from build123d import *

# Parameters (mm, degrees)
ESQUISSE1_W             = 8
ESQUISSE1_H             = 59
BOSS_EXTRU_1_DEPTH      = 60
ESQUISSE3_R             = 30
ESQUISSE3_R_2           = 29
BOSS_EXTRU_2_DEPTH      = 60
ESQUISSE4_R             = 29
ENL_V_MAT_EXTRU_3_DEPTH = 30
ENL_V_MAT_EXTRU_5_DEPTH = 1.5
ESQUISSE6_R             = 29
ENL_V_MAT_EXTRU_6_DEPTH = 22
ESQUISSE7_R             = 2
ENL_V_MAT_EXTRU_7_DEPTH = 6.5
ESQUISSE9_R             = 0.5
ENL_V_MAT_EXTRU_8_DEPTH = 4


with BuildPart() as part:
    # Esquisse1 → Boss.-Extru.1 (new body)
    with BuildSketch(Plane.XY):
        with Locations((4, 29.5)):
            Rectangle(ESQUISSE1_W, ESQUISSE1_H)
    extrude(amount=BOSS_EXTRU_1_DEPTH)

    # Esquisse3 → Boss.-Extru.2 (add)
    with BuildSketch(Plane(origin=(0, 0, 0), x_dir=(-1, 0, 0), z_dir=(0, 0, -1))):
        with Locations((-4, 29.5)):
            Circle(ESQUISSE3_R)
        with Locations((-4, 29.5)):
            Circle(ESQUISSE3_R_2, mode=Mode.SUBTRACT)
    extrude(amount=-BOSS_EXTRU_2_DEPTH)

    # Esquisse4 → Enlèv. mat.-Extru.3 (cut)
    with BuildSketch(Plane(origin=(0, 0, 0), x_dir=(-1, 0, 0), z_dir=(0, 0, -1))):
        with Locations((-4, 29.5)):
            Circle(ESQUISSE4_R)
    extrude(amount=-ENL_V_MAT_EXTRU_3_DEPTH, mode=Mode.SUBTRACT)

    # Esquisse5 → Enlèv. mat.-Extru.5 (cut)
    with BuildSketch(Plane(origin=(0, 0, 30), x_dir=(-1, 0, 0), z_dir=(0, 0, -1))):
        with BuildLine():
            Line((-6, 43), (-6.967257844, 29.9420191))
            ThreePointArc((-6.967257844, 29.9420191), (-7, 29.5), (-6.967257844, 29.0579809))
            Line((-6.967257844, 29.0579809), (-6, 16))
            ThreePointArc((-6, 16), (-4, 14), (-2, 16))
            Line((-2, 16), (-1.032742156, 29.0579809))
            ThreePointArc((-1.032742156, 29.0579809), (-1, 29.5), (-1.032742156, 29.9420191))
            Line((-1.032742156, 29.9420191), (-2, 43))
            ThreePointArc((-2, 43), (-4, 45), (-6, 43))
        make_face()
    extrude(amount=-ENL_V_MAT_EXTRU_5_DEPTH, mode=Mode.SUBTRACT)

    # Esquisse6 → Enlèv. mat.-Extru.6 (cut)
    with BuildSketch(Plane.XY.offset(60)):
        with Locations((4, 29.5)):
            Circle(ESQUISSE6_R)
    extrude(amount=-ENL_V_MAT_EXTRU_6_DEPTH, mode=Mode.SUBTRACT)

    # Esquisse7 → Enlèv. mat.-Extru.7 (cut)
    with BuildSketch(Plane(origin=(0, 0, 31.5), x_dir=(-1, 0, 0), z_dir=(0, 0, -1))):
        with Locations((-4, 29.5)):
            Circle(ESQUISSE7_R)
    extrude(amount=-ENL_V_MAT_EXTRU_7_DEPTH, mode=Mode.SUBTRACT)

    # Esquisse9 → Enlèv. mat.-Extru.8 (cut)
    with BuildSketch(Plane(origin=(0, 0, 31.5), x_dir=(-1, 0, 0), z_dir=(0, 0, -1))):
        with Locations((-4, 43)):
            Circle(ESQUISSE9_R)
        with Locations((-4, 16)):
            Circle(ESQUISSE9_R)
    extrude(amount=-ENL_V_MAT_EXTRU_8_DEPTH, mode=Mode.SUBTRACT)


solid = part.part
Build history of the part. All positions in model axes, mm. A direction names the side the tool comes from. Give positions to 0.01 mm unless a question says otherwise; leave off trailing zeros. Order: outer loops, then holes, each group sorted by start corner. A loop starts at its lowest first (then second) coordinate and runs counter-clockwise, first axis right, second up. Notation, with made-up numbers: M 75.25,9.25 L 107.25,9.25 A6 ccw 107.25,16.25 Z; hole C 64,38.25 d10. An arc over 180 degrees is marked long. Use one line per item in the form item = value.
1) Tool access for faces 1 (the face through (6.7, 29.7, 31.5)), 2 (the face through (29, 45, 60)), 3 (the face through (7, 30, 38)): list every direction of +Z, -Z, +X, -X, +Y, -Y with a clear straight run to the whole face (end or side of a thin tool).
Calculated:
face_1 = -Z
face_2 = +Z, +X, -X, +Y, -Y
face_3 = +Z
2) Saw through at B-B (y = 7.5). Give the cut face in (x, z).
Calculated:
outline = M -16.4,0 L -14.89,0 L -14.89,60 L -16.4,60 Z; M 0,30 L 8,30 L 8,38 L 0,38 Z; M 22.89,0 L 24.4,0 L 24.4,60 L 22.89,60 Z
3) Drop flat-ended pins along their axis: pin 1 (2 mm diameter, centred on x = -6.5, z = 29.5, fed in from +Y); pin 2 (1 mm diameter, centred on x = 26, z = 13.5, fed in from -Y); pin 3 (4 mm diameter, centred on x = 5, y = 20.5, fed in from -Z). Give the stop position or say it passes through.
Calculated:
pin_1 = 57.96
pin_2 = 8.58
pin_3 = 30
4) Saw through at C-C (z = 39.5). Give the cut face in (x, y), plus the area to 3 significant figures.
Calculated:
outline = C 4,29.5 d60; hole C 4,29.5 d58
area = 185 mm2
5) Two-plate mould, pull along Y, no slides. Class faces 4 (the face through (0, 29, 34)), 5 (the face through (8, 29, 34)), 6 (the face through (29, 45, 0)), 7 (the face through (-9.843, 2.885, 29.58)): released by +Y, released by -Y, zero draft, split by the parting line, or undercut.
Calculated:
face_4 = undercut
face_5 = undercut
face_6 = zero draft
face_7 = split by the parting line
6) Probe probe 1 along Y at (x, z) = (4, 32); probe 2 along Y at (x, z) = (4, 20); probe 3 along Y at (x, z) = (4, 36.75). List the from-to ranges inside material, lowest first.
Calculated:
probe_1 = -0.5 to 15.5, 16.5 to 27.5, 31.5 to 42.5, 43.5 to 59.5
probe_2 = -0.5 to 0.5, 58.5 to 59.5
probe_3 = -0.5 to 27.5, 31.5 to 59.5
7) Saw through at A-A (x = 12.5). Give the cut face in (y, z).
Calculated:
outline = M 0.73,0 L 1.77,0 L 1.77,60 L 0.73,60 Z; M 57.23,0 L 58.27,0 L 58.27,60 L 57.23,60 Z
